from build123d import *

# Parameters (mm, degrees)
ESQUISSE1_W             = 70
ESQUISSE1_H             = 12
BOSS_EXTRU_1_DEPTH      = 80
ESQUISSE2_W             = 12
ESQUISSE2_H             = 6
ENL_V_MAT_EXTRU_1_DEPTH = 107.976632963
ESQUISSE4_R             = 2.25
ENL_V_MAT_EXTRU_3_DEPTH = 107.976632963
ESQUISSE5_W             = 12
ESQUISSE5_H             = 10
BOSS_EXTRU_2_DEPTH      = 6
CHANFREIN1_SIZE         = 3
ESQUISSE6_R             = 1
ENL_V_MAT_EXTRU_4_DEPTH = 12


with BuildPart() as part:
    # Esquisse1 → Boss.-Extru.1 (new body)
    with BuildSketch(Plane.XY):
        with Locations((35, 6)):
            Rectangle(ESQUISSE1_W, ESQUISSE1_H)
    extrude(amount=BOSS_EXTRU_1_DEPTH)

    # Esquisse2 → Enlèv. mat.-Extru.1 (cut, through all)
    with BuildSketch(Plane.XY.offset(80)):
        with Locations((52.5, 9)):
            Rectangle(ESQUISSE2_W, ESQUISSE2_H)
        with Locations((17.5, 9)):
            Rectangle(ESQUISSE2_W, ESQUISSE2_H)
    extrude(amount=-ENL_V_MAT_EXTRU_1_DEPTH, mode=Mode.SUBTRACT)

    # Esquisse4 → Enlèv. mat.-Extru.3 (cut, through all)
    with BuildSketch(Plane(origin=(0, 12, 0), x_dir=(1, 0, 0), z_dir=(0, 1, 0))):
        with Locations(Location((5, -10, 0), (0, 0, 270))):
            Circle(ESQUISSE4_R)
        with Locations(Location((65, -70, 0), (0, 0, 270))):
            Circle(ESQUISSE4_R)
        with Locations(Location((65, -10, 0), (0, 0, 90))):
            Circle(ESQUISSE4_R)
        with Locations(Location((5, -70, 0), (0, 0, 90))):
            Circle(ESQUISSE4_R)
        with Locations(Location((35, -10, 0), (0, 0, 270))):
            Circle(ESQUISSE4_R)
        with Locations(Location((35, -70, 0), (0, 0, 270))):
            Circle(ESQUISSE4_R)
    extrude(amount=-ENL_V_MAT_EXTRU_3_DEPTH, mode=Mode.SUBTRACT)

    # Esquisse5 → Boss.-Extru.2 (add)
    with BuildSketch(Plane(origin=(0, 12, 0), x_dir=(1, 0, 0), z_dir=(0, 1, 0))):
        with Locations((17.5, -75)):
            Rectangle(ESQUISSE5_W, ESQUISSE5_H)
        with Locations((52.5, -75)):
            Rectangle(ESQUISSE5_W, ESQUISSE5_H)
        with Locations((52.5, -5)):
            Rectangle(ESQUISSE5_W, ESQUISSE5_H)
        with Locations((17.5, -5)):
            Rectangle(ESQUISSE5_W, ESQUISSE5_H)
    extrude(amount=-BOSS_EXTRU_2_DEPTH)

    # Chanfrein1
    chanfrein1_edges = [part.edges().sort_by_distance(p)[0] for p in [
        (70, 6, 80),
        (0, 6, 80),
        (70, 6, 0),
        (0, 6, 0),
    ]]
    chamfer(chanfrein1_edges, length=CHANFREIN1_SIZE)

    # Esquisse6 → Enlèv. mat.-Extru.4 (cut)
    with BuildSketch(Plane(origin=(0, 12, 0), x_dir=(1, 0, 0), z_dir=(0, 1, 0))):
        with Locations(Location((5, -20, 0), (0, 0, 270))):
            Circle(ESQUISSE6_R)
        with Locations(Location((5, -60, 0), (0, 0, 90))):
            Circle(ESQUISSE6_R)
        with Locations(Location((65, -60, 0), (0, 0, 270))):
            Circle(ESQUISSE6_R)
        with Locations(Location((65, -20, 0), (0, 0, 90))):
            Circle(ESQUISSE6_R)
    extrude(amount=-ENL_V_MAT_EXTRU_4_DEPTH, mode=Mode.SUBTRACT)


solid = part.part
Verification items for the finished model (mm, model axes). A direction names the side the tool comes from. Coordinates: 2 decimals unless noted, no trailing zeros. Write each loop counter-clockwise with the first axis right and the second up, starting at its lowest first coordinate (ties: lowest second). Pieces come first, ordered by that corner, then holes. Notation, with made-up numbers: M 54,-13 L 96,-13 A19 cw 96,-4 Z; hole C 12,86.5 d10. An arc over 180 degrees is marked long. Use CSV: the item, a comma, the result in double quotes.
Q1. Mould release check, pull along X, two halves, no side actions. Record for faces 1 (the cylindrical face through (67.196, 6.084, 10.488)), 2 (the flat face through (35, 6, 0)), 3 (the flat face through (70, 6, 39)): pulls with the +X half, pulls with the -X half, needs draft (parallel to the pull), parting line crosses it, or undercut.
Computed values:
face 1,"undercut"
face 2,"needs draft"
face 3,"pulls with the +X half"
Q2. Go/stop test with flat-tipped pins: P1, Ø6, axis at x = 19.5, z = 34.5, coming from the +Y side; P2, Ø1.8, axis at x = 65, z = 20, coming from the -Y side. Record where each tip stops, or that it passes through.
Computed values:
P1,"y = 6"
P2,"through"
Q3. Section check B-B, the plane y = 2.5. State how many separate pieces and enclosed holes the cut face has, and give its area (3 significant figures).
Computed values:
separate pieces,"1"
enclosed holes,"10"
area,"5,470 mm²"
Q4. Section check C-C, the plane x = 5. Enter the section's corners in (y, z).
Computed values:
outline,"M 0,0 L 12,0 L 12,7.75 L 0,7.75 Z; M 0,12.25 L 12,12.25 L 12,19 L 0,19 Z; M 0,21 L 12,21 L 12,59 L 0,59 Z; M 0,61 L 12,61 L 12,67.75 L 0,67.75 Z; M 0,72.25 L 12,72.25 L 12,80 L 0,80 Z"
Q5. Thickness scan on line 1 along X through (y, z) = (6.25, 20); line 2 along X through (y, z) = (3.5, 10); line 3 along X through (y, z) = (9.75, 46). Record the ranges inside material, lowest first. Write a range as [from, to].
Computed values:
line 1,"[0, 4], [6, 11.5], [23.5, 46.5], [58.5, 64], [66, 70]"
line 2,"[0, 2.75], [7.25, 32.75], [37.25, 62.75], [67.25, 70]"
line 3,"[0, 11.5], [23.5, 46.5], [58.5, 70]"
Q6. Set-up check for faces 4 (the flat face through (35, 6, 80)), 5 (the flat face through (52, 6, 40)): record each of +Z, -Z, +X, -X, +Y, -Y from which the full face is reachable in a straight line by a thin tool's end or side.
Computed values:
face 4,"+Z, +X, -X, +Y, -Y"
face 5,"+Y"
Q7. Section check A-A, the plane z = 60. Enter the section's corners in (x, y).
Computed values:
outline,"M 0,0 L 4,0 L 4,12 L 0,12 Z; M 6,0 L 64,0 L 64,12 L 58.5,12 L 58.5,6 L 46.5,6 L 46.5,12 L 23.5,12 L 23.5,6 L 11.5,6 L 11.5,12 L 6,12 Z; M 66,0 L 70,0 L 70,12 L 66,12 Z"
